Design review of the part built by this model. Coordinates are the model's own, in mm. A direction names the side the tool comes from. Round coordinates to 2 decimals unless told otherwise and drop trailing zeros. Loops run counter-clockwise (first coordinate to the right, second up) from the corner with the lowest first, then second, coordinate; pieces in that order, holes last. Notation, with made-up numbers: M 33.25,38 L 83.25,38 A18 cw 83.25,42 Z; hole C -27.5,16.5 d11. An arc over 180 degrees is marked long. One line per item, written item: value. Start each with the question number.
Item 1: Clearance check with flat-ended pins moving along their axes: pin 1 (2.5 mm diameter, centred on x = 0, y = -8.5, fed in from -Z); pin 2 (1.5 mm diameter, centred on x = -2, z = -2.5, fed in from -Y); pin 3 (1.5 mm diameter, centred on x = 16, z = -2, fed in from +Y); pin 4 (1.5 mm diameter, centred on y = 10, z = -1, fed in from +X). State where each tip first meets the part, or that it passes through.
Item 2: We need section A-A (x = -20). Write out the cut boundary in (y, z).
Item 3: For line 1 along Y through (x, z) = (0, 0.7); line 2 along Y through (x, z) = (20, 1.6); line 3 along Y through (x, z) = (1, -4.5), list the stretches that pass through material, from the lowest coordinate up.
Item 4: We need section C-C (y = 4.5). Write out the cut boundary in (x, z), then the cut area to 3 significant figures.
Item 5: For faces 1 (the flat face through (-17.5, 3, -2)), 2 (the flat face through (17.5, 3, -2)), 3 (the flat face through (0, 10.5, -2)), 4 (the flat face through (-23.25, 11, 4)), list the 3-axis set-ups (+Z, -Z, +X, -X, +Y, -Y) from which the entire face can be reached by the end or side of a thin tool; tool diameter is ignored.
Item 6: We need section B-B (z = 1.5). Write out the cut boundary in (x, y).
Item 7: We need section D-D (y = -7.5). Write out the cut boundary in (x, z), then the cut area to 3 significant figures.
Item 8: Mouldability with a two-part tool opening along X and no side actions: class faces 5 (the flat face through (0, 0, 5)), 6 (the flat face through (3.25, -11, 4)), 7 (the flat face through (26, 0, 2)) as released by +X, released by -X, zero draft, split by the parting line, or undercut.
from build123d import *

# Parameters (mm, degrees)
SKETCH_1_W          = 52
SKETCH_1_H          = 25
EXTRUDE_1_DEPTH     = 5
CHAMFER_1_SIZE      = 2
SKETCH_2_W          = 35
SKETCH_2_H          = 15
EXTRUDE_2_DEPTH     = 5
CUT_EXTRUDE_1_DEPTH = 3
SKETCH_5_R          = 1.6
CUT_EXTRUDE_2_DEPTH = 8


with BuildPart() as part:
    # Эскиз1 → Бобышка-Вытянуть1 (new body)
    with BuildSketch(Plane.XY):
        Rectangle(SKETCH_1_W, SKETCH_1_H)
    extrude(amount=EXTRUDE_1_DEPTH)

    # Фаска1
    chamfer_1_edges = [part.edges().sort_by_distance(p)[0] for p in [
        (26, -12.5, 2.5),
        (-26, -12.5, 2.5),
        (-26, 12.5, 2.5),
        (26, 12.5, 2.5),
    ]]
    chamfer(chamfer_1_edges, length=CHAMFER_1_SIZE)

    # Эскиз2 → Бобышка-Вытянуть2 (add)
    with BuildSketch(Plane(origin=(0, 0, 0), x_dir=(-1, 0, 0), z_dir=(0, 0, -1))):
        with Locations((0, 3)):
            Rectangle(SKETCH_2_W, SKETCH_2_H)
    extrude(amount=EXTRUDE_2_DEPTH)

    # Эскиз3 → Вырез-Вытянуть1 (cut)
    with BuildSketch(Plane.XY.offset(5)):
        with BuildLine():
            Line((3.25, -12.5), (3.25, -8.5))
            ThreePointArc((3.25, -8.5), (0, -5.25), (-3.25, -8.5))
            Line((-3.25, -8.5), (-3.25, -12.5))
            Line((-3.25, -12.5), (3.25, -12.5))
        make_face()
        with BuildLine():
            Line((-23.25, 12.5), (-23.25, 8.5))
            ThreePointArc((-23.25, 8.5), (-20, 5.25), (-16.75, 8.5))
            Line((-16.75, 8.5), (-16.75, 12.5))
            Line((-16.75, 12.5), (-23.25, 12.5))
        make_face()
        with BuildLine():
            Line((16.75, 12.5), (16.75, 8.5))
            ThreePointArc((16.75, 8.5), (20, 5.25), (23.25, 8.5))
            Line((23.25, 8.5), (23.25, 12.5))
            Line((23.25, 12.5), (16.75, 12.5))
        make_face()
    extrude(amount=-CUT_EXTRUDE_1_DEPTH, mode=Mode.SUBTRACT)

    # Эскиз5 → Вырез-Вытянуть2 (cut, through all)
    with BuildSketch(Plane.XY.offset(2)):
        with Locations((0, -8.5)):
            Circle(SKETCH_5_R)
        with Locations((-20, 8.5)):
            Circle(SKETCH_5_R)
        with Locations((20, 8.5)):
            Circle(SKETCH_5_R)
    extrude(amount=-CUT_EXTRUDE_2_DEPTH, mode=Mode.SUBTRACT)


solid = part.part
A:
1. pin 1: through
1. pin 2: y = -4.5
1. pin 3: y = 10.5
1. pin 4: x = 17.5
2. outline: M -12.5,0 L 6.9,0 L 6.9,2 L 5.25,2 L 5.25,5 L -12.5,5 Z; M 10.1,0 L 12.5,0 L 12.5,2 L 10.1,2 Z
3. line 1: -12.5 to -10.1, -6.9 to 12.5
3. line 2: -12.5 to 6.9, 10.1 to 12.5
3. line 3: -4.5 to 10.5
4. outline: M -26,0 L -17.5,0 L -17.5,-5 L 17.5,-5 L 17.5,0 L 26,0 L 26,5 L -26,5 Z
4. area: 435 mm2
5. face 1: -Z, -X, +Y, -Y
5. face 2: -Z, +X, +Y, -Y
5. face 3: -Z, +X, -X, +Y
5. face 4: +Z, +Y
6. outline: M -26,-10.5 L -24,-12.5 L 24,-12.5 L 26,-10.5 L 26,10.5 L 24,12.5 L -24,12.5 L -26,10.5 Z; hole C -20,8.5 d3.2; hole C 0,-8.5 d3.2; hole C 20,8.5 d3.2
7. outline: M -26,0 L -1.25,0 L -1.25,2 L -3.09,2 L -3.09,5 L -26,5 Z; M 1.25,0 L 26,0 L 26,5 L 3.09,5 L 3.09,2 L 1.25,2 Z
7. area: 236 mm2
8. face 5: zero draft
8. face 6: undercut
8. face 7: released by +X
